Input: dimensioned drawing with shaded views. Units: mm. Origin: part minimum x, y, z. A direction names the side the tool comes from. Coordinates: 2 decimals unless noted, no trailing zeros. Order: outer loops, then holes, each group sorted by start corner. A loop starts at its lowest first (then second) coordinate and runs counter-clockwise, first axis right, second up. Notation, with made-up numbers: (68, -34.5) -> (91, -34.5) arc R21 cw to (91, -8.5) -> close; hole circle Ø9 at (77, 24). An arc over 180 degrees is marked (long way). Answer as CSV lines item,"result".
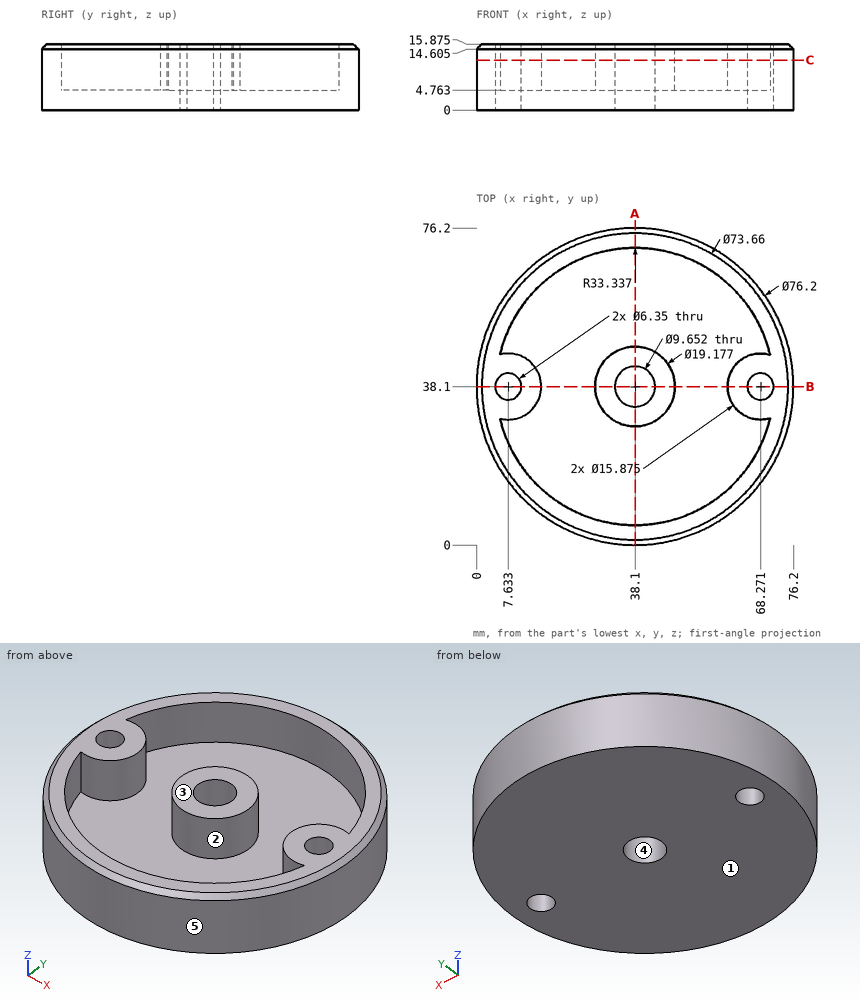
1. Cut plane C-C (z = 12). State how many separate pieces and enclosed holes the cut face has, plus the area to 3 significant figures.
Findings:
separate pieces,"2"
enclosed holes,"4"
area,"1,500 mm2"
2. Reachability of the marked faces 1 and 2 from +Z, -Z, +X, -X, +Y, -Y: full face, straight path, thin tool, end or side. Return the list, or none.
Findings:
face 1,"-Z, +X, -X, +Y, -Y"
face 2,"+Z"
3. Mould query, pull axis X, two halves, no side actions, for the marked faces 3, 4 and 5. Classes: released by +X, released by -X, zero draft, split by the parting line, or undercut.
Findings:
face 3,"zero draft"
face 4,"undercut"
face 5,"split by the parting line"
4. Contact query for flat-ended pins moving along their axis: pin 1 (8 mm diameter, centred on y = 19, z = 12, fed in from -X); pin 2 (2 mm diameter, centred on y = 58.5, z = 3, fed in from -X); pin 3 (4 mm diameter, centred on y = 22.5, z = 14, fed in from +X); pin 4 (5 mm diameter, centred on x = 7.63, y = 38.1, fed in from -Z). Output: stop coordinate, or through.
Findings:
pin 1,"stops at x = 3.12"
pin 2,"stops at x = 5.31"
pin 3,"stops at x = 73.69"
pin 4,"passes through"
5. Cut plane A-A (x = 38.1). Return the cut outline in (y, z) (1 decimal).
Findings:
outline,"(0, 0) -> (33.3, 0) -> (33.3, 15.9) -> (28.5, 15.9) -> (28.5, 4.8) -> (4.8, 4.8) -> (4.8, 15.9) -> (1.3, 15.9) -> (0, 14.6) -> close; (42.9, 0) -> (76.2, 0) -> (76.2, 14.6) -> (74.9, 15.9) -> (71.4, 15.9) -> (71.4, 4.8) -> (47.7, 4.8) -> (47.7, 15.9) -> (42.9, 15.9) -> close"
6. Ray query, line 1 along Y through (x, z) = (38.1, 12) (1 decimal); line 2 along Y through (x, z) = (61.5, 14.75) (1 decimal); line 3 along Y through (x, z) = (39, 15) (1 decimal). Return the intervals inside material, ascending.
Findings:
line 1,"y = 0 to 4.8, 28.5 to 33.3, 42.9 to 47.7, 71.4 to 76.2"
line 2,"y = 8.2 to 14.4, 34 to 42.2, 61.8 to 68"
line 3,"y = 0.4 to 4.8, 28.6 to 33.4, 42.8 to 47.6, 71.4 to 75.8"
7. Cut plane B-B (y = 38.1). Return the cut outline in (x, z) (1 decimal), plus the area to 3 significant figures.
Findings:
outline,"(0, 0) -> (4.5, 0) -> (4.5, 15.9) -> (1.3, 15.9) -> (0, 14.6) -> close; (10.8, 0) -> (33.3, 0) -> (33.3, 15.9) -> (28.5, 15.9) -> (28.5, 4.8) -> (15.6, 4.8) -> (15.6, 15.9) -> (10.8, 15.9) -> close; (42.9, 0) -> (65.1, 0) -> (65.1, 15.9) -> (60.3, 15.9) -> (60.3, 4.8) -> (47.7, 4.8) -> (47.7, 15.9) -> (42.9, 15.9) -> close; (71.4, 0) -> (76.2, 0) -> (76.2, 14.6) -> (74.9, 15.9) -> (71.4, 15.9) -> close"
area,"569 mm2"
